Read the model definition and answer for the solid it produces. Units are mm, in the model's axes. Face numbers are marked on the shaded views. A direction names the side the tool comes from. Coordinates: 2 decimals unless noted, no trailing zeros. Loops run counter-clockwise (first coordinate to the right, second up) from the corner with the lowest first, then second, coordinate; pieces in that order, holes last. Notation, with made-up numbers: (-40, 69.5) -> (-10, 69.5) arc R15 cw to (-10, 79.5) -> close; hole circle Ø4 at (40.25, 9.5). An arc over 180 degrees is marked (long way). Answer as CSV lines item,"result".
```python
from build123d import *

# Parameters (mm, degrees)
SKETCH_W        = 60
SKETCH_H        = 60
SKETCH_W_2      = 54
SKETCH_H_2      = 54
PAD_DEPTH       = 200
SKETCH001_R     = 2.75
POCKET_DEPTH    = 3
SKETCH002_R     = 2.75
POCKET001_DEPTH = 3


with BuildPart() as part:
    # Sketch → Pad (new body)
    with BuildSketch(Plane.XY):
        Rectangle(SKETCH_W, SKETCH_H)
        Rectangle(SKETCH_W_2, SKETCH_H_2, mode=Mode.SUBTRACT)
    extrude(amount=PAD_DEPTH)

    # Sketch001 (on Face3 of Pad) → Pocket (cut)
    with BuildSketch(Plane.XZ.offset(30)):
        with Locations((-20, 50)):
            Circle(SKETCH001_R)
        with Locations((20, 50)):
            Circle(SKETCH001_R)
        with Locations((-20, 10)):
            Circle(SKETCH001_R)
        with Locations((20, 10)):
            Circle(SKETCH001_R)
    extrude(amount=-POCKET_DEPTH, mode=Mode.SUBTRACT)

    # Sketch002 (on Face3 of Pocket) → Pocket001 (cut)
    with BuildSketch(Plane.YZ.offset(30)):
        with Locations((-20, 190)):
            Circle(SKETCH002_R)
        with Locations((19.999999, 189.989386)):
            Circle(SKETCH002_R)
        with Locations((-20.010614, 150.000001)):
            Circle(SKETCH002_R)
        with Locations((19.989384, 149.989387)):
            Circle(SKETCH002_R)
        with Locations((-20, 110.000001)):
            Circle(SKETCH002_R)
        with Locations((20, 110.000001)):
            Circle(SKETCH002_R)
        with Locations((-20, 70.000001)):
            Circle(SKETCH002_R)
        with Locations((20, 70.000001)):
            Circle(SKETCH002_R)
    extrude(amount=-POCKET001_DEPTH, mode=Mode.SUBTRACT)


solid = part.part
```
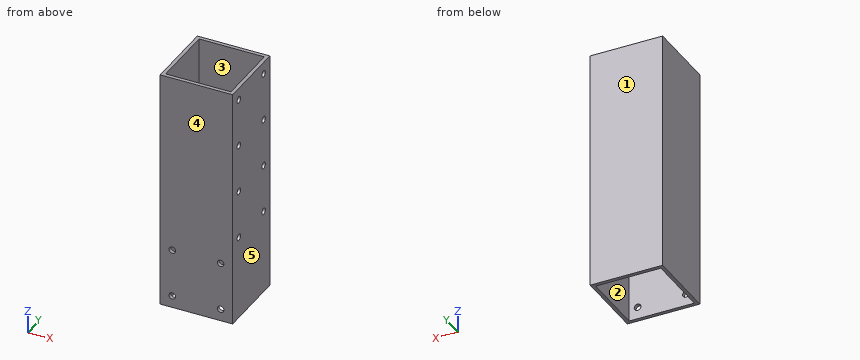
Q1. A cutting plane is placed at D-D, the plane z = 135. Write down the section's boundary in (x, y).
Results:
outline,"(-30, -30) -> (30, -30) -> (30, 30) -> (-30, 30) -> close; hole (-27, -27) -> (27, -27) -> (27, 27) -> (-27, 27) -> close"
Q2. Given pin 1 Ø4.5 at (y, z) = (20, 110) entering from +X, flat-ended and moving along its own axis, determine where the tip first touches the part or whether it passes through.
Results:
pin 1,"stops at x = -27"
Q3. A cutting plane is placed at A-A, the plane x = 15. Write down the section's boundary in (y, z).
Results:
outline,"(-30, 0) -> (-27, 0) -> (-27, 200) -> (-30, 200) -> close; (27, 0) -> (30, 0) -> (30, 200) -> (27, 200) -> close"
Q4. A cutting plane is placed at B-B, the plane z = 10. Write down the section's boundary in (x, y).
Results:
outline,"(-30, -30) -> (-22.75, -30) -> (-22.75, -27) -> (-27, -27) -> (-27, 27) -> (27, 27) -> (27, -27) -> (22.75, -27) -> (22.75, -30) -> (30, -30) -> (30, 30) -> (-30, 30) -> close; (-17.25, -30) -> (17.25, -30) -> (17.25, -27) -> (-17.25, -27) -> close"
Q5. For the marked faces 1 and 2, determine the directions among +Z, -Z, +X, -X, +Y, -Y from which every point of the face is accessible in a straight line to the end or side of a thin tool.
Results:
face 1,"+Z, -Z, +X, -X, +Y"
face 2,"+Z, -Z"
Q6. For a pull along X with two mould halves and no side action, classify the marked faces 3, 4 and 5 as pulls with the +X half, pulls with the -X half, needs draft (parallel to the pull), parting line crosses it, or undercut.
Results:
face 3,"undercut"
face 4,"needs draft"
face 5,"pulls with the +X half"
Q7. Find the intervals of material crossed by probe 1 along Z at (x, y) = (-20, -28); probe 2 along Z at (x, y) = (28.05, -20); probe 3 along Z at (x, y) = (29, 20), in increasing order. Write a range as [from, to].
Results:
probe 1,"z = [0, 7.25], [12.75, 47.25], [52.75, 200]"
probe 2,"z = [0, 67.25], [72.75, 107.25], [112.75, 147.25], [152.75, 187.25], [192.75, 200]"
probe 3,"z = [0, 67.25], [72.75, 107.25], [112.75, 147.24], [152.74, 187.24], [192.74, 200]"
